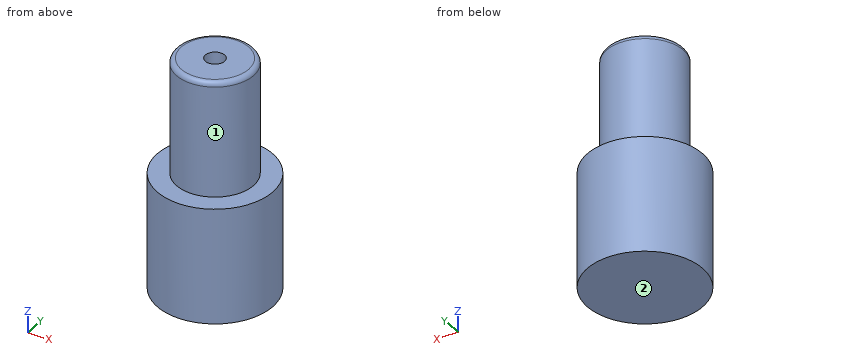
```python
from build123d import *

# Parameters (mm, degrees)
F0_R     = 1
F1_DEPTH = 2
F0_R_2   = 4
F2_DEPTH = 24
F0_R_3   = 6
F3_DEPTH = 12
F4_R     = 0.5


with BuildPart() as f1:
    # F0 (on Top) → F1 (new body)
    with BuildSketch(Plane.XY):
        Circle(F0_R)
    extrude(amount=F1_DEPTH)

    # F0 (on Top) → F2 (join)
    with BuildSketch(Plane.XY):
        Circle(F0_R_2)
        Circle(F0_R, mode=Mode.SUBTRACT)
    extrude(amount=F2_DEPTH)

    # F0 (on Top) → F3 (join)
    with BuildSketch(Plane.XY):
        Circle(F0_R_3)
        Circle(F0_R_2, mode=Mode.SUBTRACT)
    extrude(amount=F3_DEPTH)

    # F4
    f4_edges = [f1.edges().sort_by_distance(p)[0] for p in [
        (-4, 0, 24),
    ]]
    fillet(f4_edges, radius=F4_R)


solid = f1.part
```
Input: part model. Units: mm. Frame: model coordinates. Face numbers are marked on the shaded views. A direction names the side the tool comes from. Give positions to 0.01 mm unless a question says otherwise; leave off trailing zeros. Order: outer loops, then holes, each group sorted by start corner. A loop starts at its lowest first (then second) coordinate and runs counter-clockwise, first axis right, second up.
1. Section B-B on y = 0. Return the cut outline in (x, z).
Derived:
outline: (-6, 0) - (6, 0) - (6, 12) - (4, 12) - (4, 23.5) arc R0.5 ccw to (3.5, 24) - (1, 24) - (1, 2) - (-1, 2) - (-1, 24) - (-3.5, 24) arc R0.5 ccw to (-4, 23.5) - (-4, 12) - (-6, 12) - close
2. Section A-A on z = 19.75. Return the cut outline in (x, y), and give its area (3 significant figures).
Derived:
outline: circle Ø8 at (0, 0); hole circle Ø2 at (0, 0)
area: 47.1 mm2
3. Pin query (flat end, axial travel): pin 1 (1.5 mm diameter, centred on x = -4, z = 15.5, fed in from +Y); pin 2 (1.2 mm diameter, centred on x = 0, y = 0, fed in from +Z); pin 3 (4 mm diameter, centred on y = 0, z = 20, fed in from -X). Return the tip coordinate at first contact, or that it passes through.
Derived:
pin 1: stops at y = 2.33
pin 2: stops at z = 2
pin 3: stops at x = -4
4. Reachability of the marked faces 1 and 2 from +Z, -Z, +X, -X, +Y, -Y: full face, straight path, thin tool, end or side. Return the list, or none.
Derived:
face 1: +Z
face 2: -Z, +X, -X, +Y, -Y
5. Material intervals for L1, parallel to Y at x = 0, z = 9.25; L2, parallel to Y at x = 0, z = 13.75; L3, parallel to Z at x = -2, y = 5.25, sorted ascending.
Derived:
L1: y = -6 to -1, 1 to 6
L2: y = -4 to -1, 1 to 4
L3: z = 0 to 12
6. Section D-D on z = 1.75. Return the cut outline in (x, y).
Derived:
outline: circle Ø12 at (0, 0)
